Geometry: final body of the model. Coordinates: model frame, mm. A direction names the side the tool comes from. Give positions to 0.01 mm unless a question says otherwise; leave off trailing zeros. Write each loop counter-clockwise with the first axis right and the second up, starting at its lowest first coordinate (ties: lowest second). Pieces come first, ordered by that corner, then holes.
Q1. Section D-D (y = -30). Return the cut outline in (x, z), plus the area to 3 significant figures.
Q2. Pin query (flat end, axial travel): pin 1 Ø10 at (y, z) = (33.5, -29.5) entering from +X; pin 2 Ø2 at (x, y) = (7, -6) entering from -Z; pin 3 Ø22 at (x, z) = (15.5, -30.5) entering from -Y. Return the tip coordinate at first contact, or that it passes through.
Q3. Reachability of faces 4 (the flat face through (-33, -3, -36)), 5 (the flat face through (-36.55, 0.92, -33.97)), 6 (the flat face through (36.55, -4.15, -35.99)) from +Z, -Z, +X, -X, +Y, -Y: full face, straight path, thin tool, end or side. Return the list, or none.
Q4. Line query: line 1 (Y direction, x = 20, z = 3); line 2 (Y direction, x = 3.5, z = -56.5); line 3 (Z direction, x = 21.5, y = 6.5). Output: solid intervals per line, ascending.
Q5. Section C-C (y = 5). Return the cut outline in (x, z).
Q6. Section B-B (z = -58.5). Return the cut outline in (x, y), plus the area to 3 significant figures.
Q7. Section A-A (x = 23). Return the cut outline in (y, z).
Q8. Mould query, pull axis Y, two halves, no side actions, for faces 1 (the flat face through (40, 4, -39)), 2 (the flat face through (-1, 50, -34)), 3 (the flat face through (-1, -3, 0)). Classes: +Y half, -Y half, draft (parallel to the pull), parting line (faces both ways), or undercut.
from build123d import *

# Parameters (mm, degrees)
SKETCH1_W           = 80
SKETCH1_H           = 100
BOSS_EXTRUDE1_DEPTH = 7
SKETCH2_R           = 5
CUT_EXTRUDE1_DEPTH  = 7
SKETCH4_W           = 80
SKETCH4_H           = 80
BOSS_EXTRUDE2_DEPTH = 7
BOSS_EXTRUDE4_DEPTH = 7
SKETCH6_R           = 1.5
CUT_EXTRUDE2_DEPTH  = 7


with BuildPart() as part:
    # Sketch1 → Boss-Extrude1 (new body)
    with BuildSketch(Plane.XY):
        Rectangle(SKETCH1_W, SKETCH1_H)
    extrude(amount=BOSS_EXTRUDE1_DEPTH)

    # Sketch2 → Cut-Extrude1 (cut)
    with BuildSketch(Plane(origin=(0, 0, 0), x_dir=(-1, 0, 0), z_dir=(0, 0, -1))):
        with Locations((-20, 30)):
            Circle(SKETCH2_R)
        with Locations((20, 30)):
            Circle(SKETCH2_R)
        with Locations((20, -30)):
            Circle(SKETCH2_R)
        with Locations((-20, -30)):
            Circle(SKETCH2_R)
    extrude(amount=-CUT_EXTRUDE1_DEPTH, mode=Mode.SUBTRACT)

    # Sketch4 → Boss-Extrude2 (add)
    with BuildSketch(Plane(origin=(0, 50, 0), x_dir=(1, 0, 0), z_dir=(0, 1, 0))):
        with Locations((0, 33)):
            Rectangle(SKETCH4_W, SKETCH4_H)
    extrude(amount=-BOSS_EXTRUDE2_DEPTH)

    # Sketch5 → Boss-Extrude4 (add)
    with BuildSketch(Plane(origin=(40, 0, 0), x_dir=(0, 0, -1), z_dir=(1, 0, 0))):
        Polygon((0, -50), (73, 43), (67, 43), (-6, -50), align=None)
    boss_extrude4 = extrude(amount=-BOSS_EXTRUDE4_DEPTH)

    # Mirror3: Boss-Extrude4 across plane
    add(boss_extrude4.mirror(Plane(origin=(0, 0, 0), x_dir=(0, 0, 1), z_dir=(1, 0, 0))))

    # Sketch6 → Cut-Extrude2 (cut)
    with BuildSketch(Plane(origin=(0, 50, 0), x_dir=(1, 0, 0), z_dir=(0, 1, 0))):
        with Locations(Location((-17, 63, 0), (0, 0, 180))):
            Circle(SKETCH6_R)
        with Locations(Location((17, 63, 0), (0, 0, 180))):
            Circle(SKETCH6_R)
    extrude(amount=-CUT_EXTRUDE2_DEPTH, mode=Mode.SUBTRACT)


solid = part.part
Computed:
1. outline: (-40, -15.7) - (-33, -15.7) - (-33, -9.7) - (-40, -9.7) - close; (-40, 0) - (-25, 0) - (-25, 7) - (-40, 7) - close; (-15, 0) - (15, 0) - (15, 7) - (-15, 7) - close; (25, 0) - (40, 0) - (40, 7) - (25, 7) - close; (33, -15.7) - (40, -15.7) - (40, -9.7) - (33, -9.7) - close
1. area: 504 mm2
2. pin 1: passes through
2. pin 2: stops at z = 0
2. pin 3: stops at y = 43
3. face 4: -Z, -Y
3. face 5: +X, -X
3. face 6: -Z, +X, -X, -Y
4. line 1: y = -50 to -35, -25 to 25, 35 to 50
4. line 2: y = 43 to 50
4. line 3: z = 0 to 7
5. outline: (-40, -43.17) - (-33, -43.17) - (-33, -37.17) - (-40, -37.17) - close; (-40, 0) - (40, 0) - (40, 7) - (-40, 7) - close; (33, -43.17) - (40, -43.17) - (40, -37.17) - (33, -37.17) - close
6. outline: (-40, 24.53) - (-33, 24.53) - (-33, 32.17) - (-40, 32.17) - close; (-40, 43) - (40, 43) - (40, 50) - (-40, 50) - close; (33, 24.53) - (40, 24.53) - (40, 32.17) - (33, 32.17) - close
6. area: 667 mm2
7. outline: (-50, 0) - (-34, 0) - (-34, 7) - (-50, 7) - close; (-26, 0) - (26, 0) - (26, 7) - (-26, 7) - close; (34, 0) - (43, 0) - (43, -73) - (50, -73) - (50, 7) - (34, 7) - close
8. face 1: draft
8. face 2: +Y half
8. face 3: undercut
